Build history of the part. All positions in model axes, mm. Face numbers are marked on the shaded views. A direction names the side the tool comes from. Give positions to 0.01 mm unless a question says otherwise; leave off trailing zeros. Order: outer loops, then holes, each group sorted by start corner. A loop starts at its lowest first (then second) coordinate and runs counter-clockwise, first axis right, second up. Notation, with made-up numbers: M 34.5,-31.75 L 64.5,-31.75 A23 cw 64.5,6.25 Z; hole C -13,70.5 d10. An arc over 180 degrees is marked long. One line per item, written item: value.
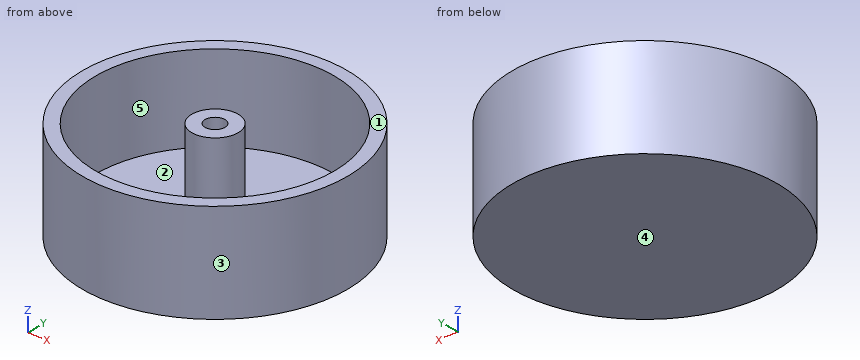
from build123d import *

# Parameters (mm, degrees)
F0_R     = 20
F1_DEPTH = 15
F2_R     = 18
F3_DEPTH = 13
F4_R     = 3.5
F4_R_2   = 1.5
F5_DEPTH = 13


with BuildPart() as f1:
    # F0 (on Top) → F1 (new body)
    with BuildSketch(Plane.XY):
        Circle(F0_R)
    extrude(amount=F1_DEPTH)

    # F2 (on face) → F3 (cut)
    with BuildSketch(Plane.XY.offset(15)):
        Circle(F2_R)
    extrude(amount=-F3_DEPTH, mode=Mode.SUBTRACT)

    # F4 (on face) → F5 (join)
    with BuildSketch(Plane.XY.offset(2)):
        Circle(F4_R)
        Circle(F4_R_2, mode=Mode.SUBTRACT)
    extrude(amount=F5_DEPTH)


solid = f1.part
1) Mould opens along X. For the marked faces 3, 4 and 5 say: released by +X, released by -X, zero draft, split by the parting line, or undercut.
Check values:
face 3: split by the parting line
face 4: zero draft
face 5: undercut
2) Saw through at B-B, the plane y = 0. Write the cut outline in (x, z).
Check values:
outline: M -20,0 L 20,0 L 20,15 L 18,15 L 18,2 L 3.5,2 L 3.5,15 L 1.5,15 L 1.5,2 L -1.5,2 L -1.5,15 L -3.5,15 L -3.5,2 L -18,2 L -18,15 L -20,15 Z
3) Saw through at D-D, the plane x = 7. Write the cut outline in (y, z) (3 decimals).
Check values:
outline: M -18.735,0 L 18.735,0 L 18.735,15 L 16.583,15 L 16.583,2 L -16.583,2 L -16.583,15 L -18.735,15 Z
4) Saw through at A-A, the plane z = 6.5. Write the cut outline in (x, y), then the cut area to 3 significant figures.
Check values:
outline: C 0,0 d40; C 0,0 d7; hole C 0,0 d36; hole C 0,0 d3
area: 270 mm^2
5) Tool access for the marked faces 1 and 2: list every direction of +Z, -Z, +X, -X, +Y, -Y with a clear straight run to the whole face (end or side of a thin tool).
Check values:
face 1: +Z, +X, -X, +Y, -Y
face 2: +Z
6) Drill centre lines: probe 1 along Y at (x, z) = (3, 12); probe 2 along Y at (x, z) = (0, 6.5); probe 3 along Z at (x, y) = (-6.5, 1). Where is each one in solid material? Low to high. Write a range as from..to.
Check values:
probe 1: -19.77..-17.75, -1.8..1.8, 17.75..19.77
probe 2: -20..-18, -3.5..-1.5, 1.5..3.5, 18..20
probe 3: 0..2
7) Pin check, flat tips, straight feed: pin 1 (5 mm diameter, centred on y = 14.5, z = 11.5, fed in from +X); pin 2 (1 mm diameter, centred on x = -6.5, z = 10, fed in from -Y); pin 3 (1.5 mm diameter, centred on x = -12.5, y = -9.5, fed in from +Z). Stop position of each tip, or through.
Check values:
pin 1: x = 16
pin 2: y = -19.08
pin 3: z = 2
